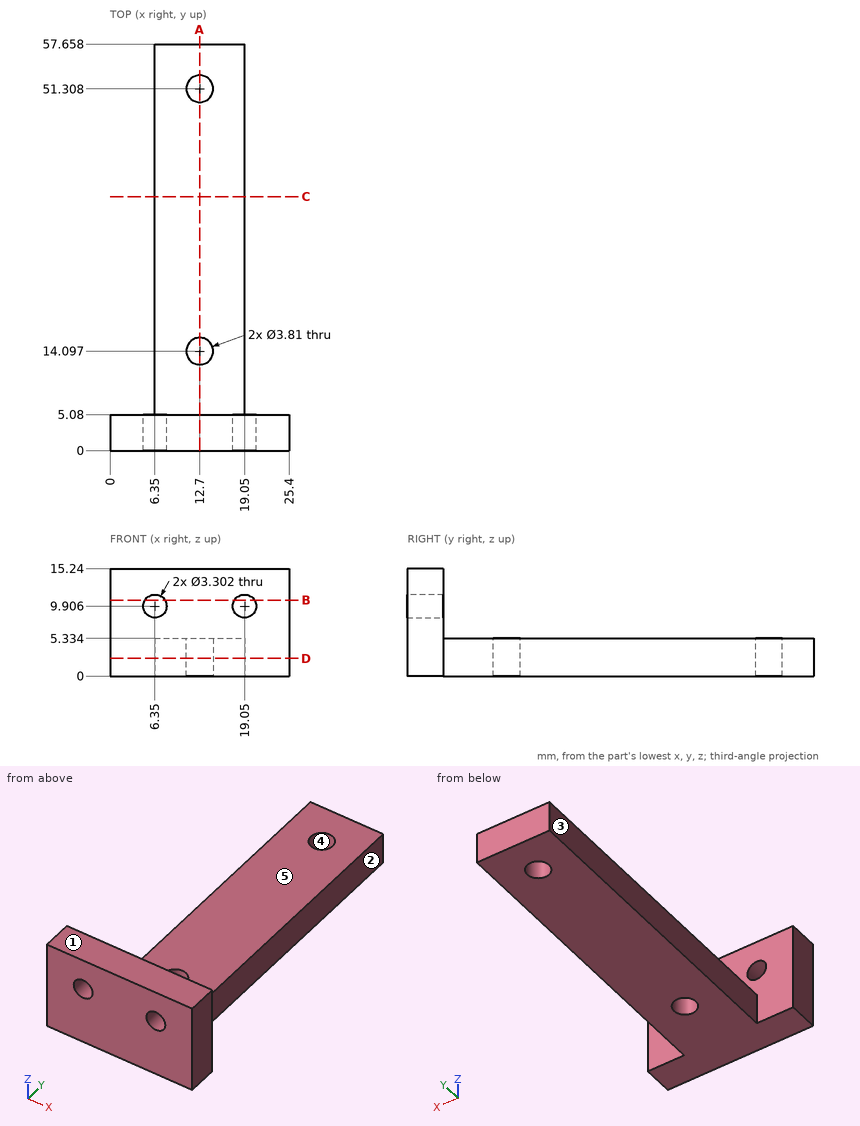
Verification items for this drawing (mm, ordinates from the low corner). A direction names the side the tool comes from. Give positions to 0.01 mm unless a question says otherwise; leave off trailing zeros. Write each loop counter-clockwise with the first axis right and the second up, starting at its lowest first coordinate (ties: lowest second). Pieces come first, ordered by that corner, then holes. Notation, with made-up numbers: (67, -28) - (121, -28) arc R8 ccw to (121, -18) - close; hole circle Ø5 at (-16, -36). An arc over 180 degrees is marked (long way). Answer as CSV lines item,"result". Start each with the question number.
1. Sectioned sample at B-B (z = 10.75). Record the boundary of the cut face in (x, y), then the cut area to 3 significant figures.
2. Draft check along X on the marked faces 3, 4 and 5. Enter one of: pulls with the +X half, pulls with the -X half, needs draft (parallel to the pull), parting line crosses it, or undercut.
3. Thickness scan on line 1 (Y direction, x = 12.7, z = 3.9); line 2 (Z direction, x = 16.75, y = 44.5); line 3 (Y direction, x = 4.75, z = 1.25). Record the ranges inside material, lowest first.
4. Sectioned sample at C-C (y = 36). Record the boundary of the cut face in (x, z).
5. Sectioned sample at D-D (z = 2.5). Record the boundary of the cut face in (x, y) (3 decimals), then the cut area to 3 significant figures.
6. Sectioned sample at A-A (x = 12.7). Record the boundary of the cut face in (y, z), then the cut area to 3 significant figures.
7. Depth check by flat-ended pin: pin 1 (1.5 mm diameter, centred on y = 6, z = 2.5, fed in from -X); pin 2 (1.6 mm diameter, centred on y = 23, z = 4, fed in from +X); pin 3 (3 mm diameter, centred on x = 10.5, y = 12.5, fed in from +Z). Enter the tip coordinate at first touch or a pass-through.
8. Set-up check for the marked faces 1 and 2: record each of +Z, -Z, +X, -X, +Y, -Y from which the full face is reachable in a straight line by a thin tool's end or side.
Derived:
1,outline,"(0, 0) - (4.93, 0) - (4.93, 5.08) - (0, 5.08) - close; (7.77, 0) - (17.63, 0) - (17.63, 5.08) - (7.77, 5.08) - close; (20.47, 0) - (25.4, 0) - (25.4, 5.08) - (20.47, 5.08) - close"
1,area,"100 mm²"
2,face 3,"pulls with the -X half"
2,face 4,"undercut"
2,face 5,"needs draft"
3,line 1,"0 to 12.19, 16 to 49.4, 53.21 to 57.66"
3,line 2,"0 to 5.33"
3,line 3,"0 to 5.08"
4,outline,"(6.35, 0) - (19.05, 0) - (19.05, 5.33) - (6.35, 5.33) - close"
5,outline,"(0, 0) - (25.4, 0) - (25.4, 5.08) - (19.05, 5.08) - (19.05, 57.658) - (6.35, 57.658) - (6.35, 5.08) - (0, 5.08) - close; hole circle Ø3.81 at (12.7, 14.097); hole circle Ø3.81 at (12.7, 51.308)"
5,area,"774 mm²"
6,outline,"(0, 0) - (12.19, 0) - (12.19, 5.33) - (5.08, 5.33) - (5.08, 15.24) - (0, 15.24) - close; (16, 0) - (49.4, 0) - (49.4, 5.33) - (16, 5.33) - close; (53.21, 0) - (57.66, 0) - (57.66, 5.33) - (53.21, 5.33) - close"
6,area,"317 mm²"
7,pin 1,"x = 6.35"
7,pin 2,"x = 19.05"
7,pin 3,"z = 5.33"
8,face 1,"+Z, +X, -X, +Y, -Y"
8,face 2,"+Z, -Z, +X, +Y"
